```python
from build123d import *

# Parameters (mm, degrees)
F0_R     = 6.85
F1_DEPTH = 7.6
F2_R     = 1.25
F3_DEPTH = 1
F4_R     = 0.35
F5_DEPTH = 5.5


with BuildPart() as f1:
    # F0 (on Top) → F1 (new body)
    with BuildSketch(Plane.XY):
        Circle(F0_R)
    extrude(amount=F1_DEPTH)

    # F2 (on face) → F3 (cut)
    with BuildSketch(Plane.XY.offset(7.6)):
        Circle(F2_R)
    extrude(amount=-F3_DEPTH, mode=Mode.SUBTRACT)

    # F4 (on face) → F5 (join)
    with BuildSketch(Plane(origin=(0, 0, 0), x_dir=(1, 0, 0), z_dir=(0, 0, -1))):
        with Locations((0, 3.81)):
            Circle(F4_R)
        with Locations((0, -3.81)):
            Circle(F4_R)
    extrude(amount=F5_DEPTH)


solid = f1.part
```
Can you work these out from the model? Positions are in its coordinate system, mm. Coordinates: 2 decimals unless noted, no trailing zeros. Loops run counter-clockwise (first coordinate to the right, second up) from the corner with the lowest first, then second, coordinate; pieces in that order, holes last. Notation, with made-up numbers: (-26, 88) -> (22, 88) arc R14 cw to (22, 111) -> close; hole circle Ø4 at (14, 59). An arc over 180 degrees is marked (long way). Put each result on its own line as item: value. Start each with the question number.
Q1. If I drill on line 1 (Y direction, x = 0, z = 6.9); line 2 (Z direction, x = 4.75, y = 1.5); line 3 (X direction, y = -3.75, z = -4.5), over which ranges is the centre line in solid material (lowest first)? Write a range as [from, to].
Q2. Thinking about a two-plate mould opening in Y: for faces 1 (the face through (-5.05, 4.63, 3.75)), 2 (the face through (0, 0, 6.6)), 3 (the face through (-0.1, -1.4, 7.6)), which applies, pulls with the +Y half, pulls with the -Y half, needs draft (parallel to the pull), parting line crosses it, or undercut?
Q3. I'm going to push flat-ended pins straight in: P1, Ø1.5, axis at x = 4, y = -1.5, coming from the -Z side; P2, Ø6, axis at x = 4.5, y = -5.5, coming from the +Z side; P3, Ø1, axis at y = 2.5, z = 2.5, coming from the +X side; P4, Ø0.8, axis at x = 0, y = 0.5, coming from the +Z side. Where does each tip first touch, or does it pass through?
Q4. I want a section at C-C (y = -1). Write out the boundary of the cut face in (x, z), plus the area to 3 significant figures.
Q5. I want a section at A-A (x = 0). Write out the boundary of the cut face in (y, z), plus the area to 3 significant figures.
Q6. I want a section at D-D (z = 5.75). Write out the boundary of the cut face in (x, y), plus the area to 3 significant figures.
Q7. I want a section at B-B (z = -4.25). Write out the boundary of the cut face in (x, y).
Taken from the geometry:
1. line 1: y = [-6.85, -1.25], [1.25, 6.85]
1. line 2: z = [0, 7.6]
1. line 3: x = [-0.34, 0.34]
2. face 1: parting line crosses it
2. face 2: undercut
2. face 3: needs draft
3. P1: stops at z = 0
3. P2: stops at z = 7.6
3. P3: stops at x = 6.55
3. P4: stops at z = 6.6
4. outline: (-6.78, 0) -> (6.78, 0) -> (6.78, 7.6) -> (0.75, 7.6) -> (0.75, 6.6) -> (-0.75, 6.6) -> (-0.75, 7.6) -> (-6.78, 7.6) -> close
4. area: 102 mm2
5. outline: (-6.85, 0) -> (-4.16, 0) -> (-4.16, -5.5) -> (-3.46, -5.5) -> (-3.46, 0) -> (3.46, 0) -> (3.46, -5.5) -> (4.16, -5.5) -> (4.16, 0) -> (6.85, 0) -> (6.85, 7.6) -> (1.25, 7.6) -> (1.25, 6.6) -> (-1.25, 6.6) -> (-1.25, 7.6) -> (-6.85, 7.6) -> close
5. area: 109 mm2
6. outline: circle Ø13.7 at (0, 0)
6. area: 147 mm2
7. outline: circle Ø0.7 at (0, -3.81); circle Ø0.7 at (0, 3.81)
